Read the model definition and answer for the solid it produces. Units are mm, in the model's axes. Coordinates: 2 decimals unless noted, no trailing zeros. Order: outer loops, then holes, each group sorted by start corner. A loop starts at its lowest first (then second) coordinate and runs counter-clockwise, first axis right, second up. Notation, with made-up numbers: M 81.5,-29 L 135.5,-29 A37 cw 135.5,8 Z; hole C 89,31 d10. An arc over 180 degrees is marked long. Use a Markdown table: item, result. Add a question column.
1) Find section B-B on y = -2.25. Write down the section's boundary in (x, z), plus the area to 3 significant figures.
2) Find the intervals of material crossed by probe 1 along Z at (x, y) = (-3.5, -1); probe 2 along X at (y, z) = (-0.25, 114); probe 3 along Z at (x, y) = (-2.5, 3), in increasing order. Write a range as [from, to].
3) Each of these flat-tipped pins is pushed along its axis until it touches: pin 1 Ø1 at (x, y) = (2.5, -1.5) entering from -Z; pin 2 Ø1 at (x, z) = (-2.5, 73.5) entering from +Y; pin 3 Ø3 at (y, z) = (-2, 96) entering from +X; pin 4 Ø3 at (x, z) = (-2, 16) entering from -Y. Where does it stop, or does it pass through?
4) Find section A-A on z = 64. Write down the section's boundary in (x, y).
from build123d import *

# Parameters (mm, degrees)
SKETCH1_R           = 4
BOSS_EXTRUDE1_DEPTH = 150
CUT_EXTRUDE1_DEPTH  = 7.5
SKETCH3_R           = 4
SKETCH3_R_2         = 3.5
CUT_EXTRUDE2_DEPTH  = 1


with BuildPart() as part:
    # Sketch1 → Boss-Extrude1 (new body)
    with BuildSketch(Plane.XY):
        Circle(SKETCH1_R)
    extrude(amount=BOSS_EXTRUDE1_DEPTH)

    # Sketch2 → Cut-Extrude1 (cut)
    with BuildSketch(Plane.XY.offset(150)):
        with BuildLine():
            Line((3.122498999, 2.5), (-3.122498999, 2.5))
            ThreePointArc((-3.122498999, 2.5), (0, 4), (3.122498999, 2.5))
        make_face()
    extrude(amount=-CUT_EXTRUDE1_DEPTH, mode=Mode.SUBTRACT)

    # Sketch3 → Cut-Extrude2 (cut)
    with BuildSketch(Plane.XY.offset(148.75)):
        Circle(SKETCH3_R)
        Circle(SKETCH3_R_2, mode=Mode.SUBTRACT)
    extrude(amount=-CUT_EXTRUDE2_DEPTH, mode=Mode.SUBTRACT)


solid = part.part
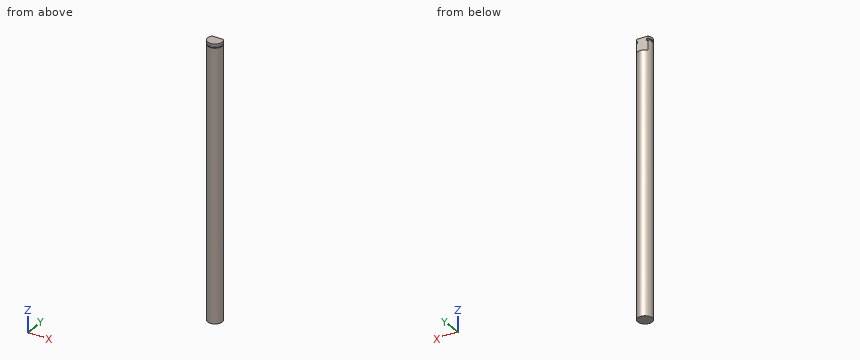
Check result:
| question | item | result |
|---|---|---|
| 1 | outline | M -3.31,0 L 3.31,0 L 3.31,147.75 L 2.68,147.75 L 2.68,148.75 L 3.31,148.75 L 3.31,150 L -3.31,150 L -3.31,148.75 L -2.68,148.75 L -2.68,147.75 L -3.31,147.75 Z |
| 1 | area | 991 mm2 |
| 2 | probe 1 | z = [0, 147.75], [148.75, 150] |
| 2 | probe 2 | x = [-3.99, 3.99] |
| 2 | probe 3 | z = [0, 142.5] |
| 3 | pin 1 | stops at z = 0 |
| 3 | pin 2 | stops at y = 3.46 |
| 3 | pin 3 | stops at x = 3.97 |
| 3 | pin 4 | stops at y = -3.97 |
| 4 | outline | C 0,0 d8 |
